Input: part model. Units: mm. Frame: model coordinates. A direction names the side the tool comes from. Round coordinates to 2 decimals unless told otherwise and drop trailing zeros. Loops run counter-clockwise (first coordinate to the right, second up) from the corner with the lowest first, then second, coordinate; pieces in that order, holes last.
(1) Cut plane A-A, the plane y = 59.5. Output: boundary loops of the cut face in (x, z), and give its area (3 significant figures).
(2) Line query: line 1 (Y direction, x = 1.9, z = -19.5); line 2 (Y direction, x = 2.5, z = -13.25); line 3 (Y direction, x = 2.25, z = -2.75). Output: solid intervals per line, ascending.
(3) Access query for faces 5 (the face through (2, 15, -11.52)), 6 (the face through (2, 54.73, -21)), 7 (the face through (2, 54.73, -3)), 8 (the face through (2, 60, -15)), 9 (the face through (2, 10, 0)). Directions: +Z, -Z, +X, -X, +Y, -Y. A direction counts if a zero-diameter tool reaches every point of the face in a straight line with its end or side. Return the directions, or none.
(4) First-contact query: pin 1 Ø1 at (x, z) = (2, -17) entering from -Y; pin 2 Ø1.6 at (x, y) = (2, 60) entering from -Z; pin 3 Ø1 at (x, y) = (2, 58) entering from +Z. Flat tips, straight axial feed; report the tip coordinate or a pass-through.
(5) Draft query along Z for faces 1 (the face through (2, 49, 0)), 2 (the face through (2, 37.811, -2)), 3 (the face through (1.57, 12.45, -22.92)), 4 (the face through (2, 12, -24.67)). Return one class per face: released by +Z, released by -Z, zero draft, split by the parting line, or undercut.
(6) Cut plane C-C, the plane y = 12.38. Output: boundary loops of the cut face in (x, z), and give its area (3 significant figures).
(7) Cut plane B-B, the plane x = 2.65. Give the number of separate pieces and of enclosed holes in the cut face, and give its area (3 significant figures).
(8) Cut plane D-D, the plane z = -21.42. Output: boundary loops of the cut face in (x, y), and give its area (3 significant figures).
from build123d import *

# Parameters (mm, degrees)
BOSS_EXTRUDE1_DEPTH     = 3.18
SKETCH2_4_OUTSIDE_W     = 40.864
SKETCH2_4_OUTSIDE_H     = 68.924
SKETCH2_4_OUTSIDE_R     = 5
CUT_EXTRUDE2_DEPTH      = 3.18
FILLET6_R               = 3
M3_5X0_6_TAPPED_HOLE1_D = 3
SKETCH9_W               = 3.18
SKETCH9_H               = 12
BOSS_EXTRUDE2_DEPTH     = 8.36
SKETCH10_W              = 6
SKETCH10_H              = 3.28
CUT_EXTRUDE3_DEPTH      = 68.81643901


with BuildPart() as part:
    # Sketch2 → Boss-Extrude1 (new body)
    with BuildSketch(Plane(origin=(0, 0, 0), x_dir=(0, 0, -1), z_dir=(1, 0, 0))):
        with BuildLine():
            Line((0, 54.73), (24, 54.73))
            Line((24, 54.73), (24, 15.53))
            Line((24, 15.53), (11.52, 15.53))
            Line((11.52, 15.53), (11.52, 14.38))
            Line((11.52, 14.38), (24.67, 14.38))
            Line((24.67, 14.38), (24.67, 10.38))
            Line((24.67, 10.38), (10.17, 10.38))
            Line((10.17, 10.38), (10.17, 0))
            Line((10.17, 0), (0, 0))
            Line((0, 0), (0, 17.7))
            Line((0, 17.7), (-2, 19.7))
            Line((-2, 19.7), (-2, 29.7))
            Line((-2, 29.7), (0, 31.7))
            Line((0, 31.7), (0, 37.810865899))
            Line((0, 37.810865899), (3.803847577, 37.810865899))
            ThreePointArc((3.803847577, 37.810865899), (15, 40.810865899), (3.803847577, 43.810865899))
            Line((3.803847577, 43.810865899), (0, 43.810865899))
            Line((0, 43.810865899), (0, 54.73))
        make_face()
    extrude(amount=-BOSS_EXTRUDE1_DEPTH)

    # Sketch2<4> outside → Cut-Extrude2 (cut)
    # profile 1 of 2: a face of its own
    with BuildSketch(Plane(origin=(0, 0, 0), x_dir=(0, 0, -1), z_dir=(1, 0, 0))):
        with Locations((11.335, 27.365)):
            Rectangle(SKETCH2_4_OUTSIDE_W, SKETCH2_4_OUTSIDE_H)
        with BuildLine():
            Line((0, 54.73), (24, 54.73))
            Line((24, 54.73), (24, 15.53))
            Line((24, 15.53), (11.52, 15.53))
            Line((11.52, 15.53), (11.52, 14.38))
            Line((11.52, 14.38), (24.67, 14.38))
            Line((24.67, 14.38), (24.67, 10.38))
            Line((24.67, 10.38), (10.17, 10.38))
            Line((10.17, 10.38), (10.17, 0))
            Line((10.17, 0), (0, 0))
            Line((0, 0), (0, 17.7))
            Line((0, 17.7), (-2, 19.7))
            Line((-2, 19.7), (-2, 29.7))
            Line((-2, 29.7), (0, 31.7))
            Line((0, 31.7), (0, 37.810865899))
            Line((0, 37.810865899), (3.803847577, 37.810865899))
            ThreePointArc((3.803847577, 37.810865899), (15, 40.810865899), (3.803847577, 43.810865899))
            Line((3.803847577, 43.810865899), (0, 43.810865899))
            Line((0, 43.810865899), (0, 54.73))
        make_face(mode=Mode.SUBTRACT)
    # profile 2 of 2: a face of its own
    with BuildSketch(Plane(origin=(0, 0, 0), x_dir=(0, 0, -1), z_dir=(1, 0, 0))):
        with Locations((5, 24.7)):
            Circle(SKETCH2_4_OUTSIDE_R)
    extrude(amount=-CUT_EXTRUDE2_DEPTH, mode=Mode.SUBTRACT)

    # Fillet6
    fillet6_edges = [part.edges().sort_by_distance(p)[0] for p in [
        (-1.59, 31.7, 0),
        (-1.59, 29.7, 2),
        (-1.59, 19.7, 2),
        (-1.59, 17.7, 0),
        (-1.59, 0, 0),
    ]]
    fillet(fillet6_edges, radius=FILLET6_R)


with BuildPart() as body_2:
    # Mirror1: mirrored copy
    add(part.part.mirror(Plane(origin=(0, 40.810865899, -9), x_dir=(0, 0, 1), z_dir=(1, 0, 0))))

    # M3.5x0.6 Tapped Hole1 (through all)
    with Locations(Plane(origin=(3.18, 0, 0), x_dir=(0, 0, -1), z_dir=(1, 0, 0))):
        with Locations((21.42, 12.38), (14.92, 12.38)):
            Hole(M3_5X0_6_TAPPED_HOLE1_D / 2)

    # Sketch9 → Boss-Extrude2 (add)
    with BuildSketch(Plane(origin=(0, 54.73, 0), x_dir=(1, 0, 0), z_dir=(0, 1, 0))):
        with Locations((1.59, 12)):
            Rectangle(SKETCH9_W, SKETCH9_H)
    extrude(amount=BOSS_EXTRUDE2_DEPTH)

    # Sketch10 → Cut-Extrude3 (cut, through all)
    with BuildSketch(Plane(origin=(3.18, 0, 0), x_dir=(0, 0, -1), z_dir=(1, 0, 0))):
        with Locations((12, 59.55)):
            Rectangle(SKETCH10_W, SKETCH10_H)
    extrude(amount=-CUT_EXTRUDE3_DEPTH, mode=Mode.SUBTRACT)


solid = body_2.part
Reported:
1. outline: (0, -18) - (3.18, -18) - (3.18, -15) - (0, -15) - close; (0, -9) - (3.18, -9) - (3.18, -6) - (0, -6) - close
1. area: 19.1 mm2
2. line 1: y = 10.38 to 14.38, 15.53 to 54.73
2. line 2: y = 10.38 to 14.38, 15.53 to 36.58, 45.05 to 57.91, 61.19 to 63.09
2. line 3: y = 0.01 to 20.23, 29.17 to 37.81, 43.81 to 54.73
3. face 5: -Z, +X, -X
3. face 6: -Z, +X, -X, +Y
3. face 7: +Z, +X, -X, +Y
3. face 8: +X, -X
3. face 9: +Z, +X, -X, -Y
4. pin 1: stops at y = 10.38
4. pin 2: stops at z = -18
4. pin 3: stops at z = -6
5. face 1: released by +Z
5. face 2: zero draft
5. face 3: undercut
5. face 4: released by -Z
6. outline: (0, -24.67) - (3.18, -24.67) - (3.18, -22.92) - (0, -22.92) - close; (0, -19.92) - (3.18, -19.92) - (3.18, -16.42) - (0, -16.42) - close; (0, -13.42) - (3.18, -13.42) - (3.18, 0) - (0, 0) - close
6. area: 59.4 mm2
7. separate pieces: 1
7. enclosed holes: 4
7. area: 1,040 mm2
8. outline: (0, 10.38) - (3.18, 10.38) - (3.18, 10.88) - (0, 10.88) - close; (0, 13.88) - (3.18, 13.88) - (3.18, 14.38) - (0, 14.38) - close; (0, 15.53) - (3.18, 15.53) - (3.18, 54.73) - (0, 54.73) - close
8. area: 128 mm2
